The drawing under review shows one solid part. Ordinate dimensions are in mm from its lowest x, y, z. Coordinates: 2 decimals unless noted, no trailing zeros. Order: outer loops, then holes, each group sorted by start corner. A loop starts at its lowest first (then second) coordinate and runs counter-clockwise, first axis right, second up. Notation, with made-up numbers: M 47.5,-18.5 L 79.5,-18.5 A14 cw 79.5,-7.5 Z; hole C 12,44 d3. An arc over 180 degrees is marked long. Answer as a JSON object with one key per item and string values.
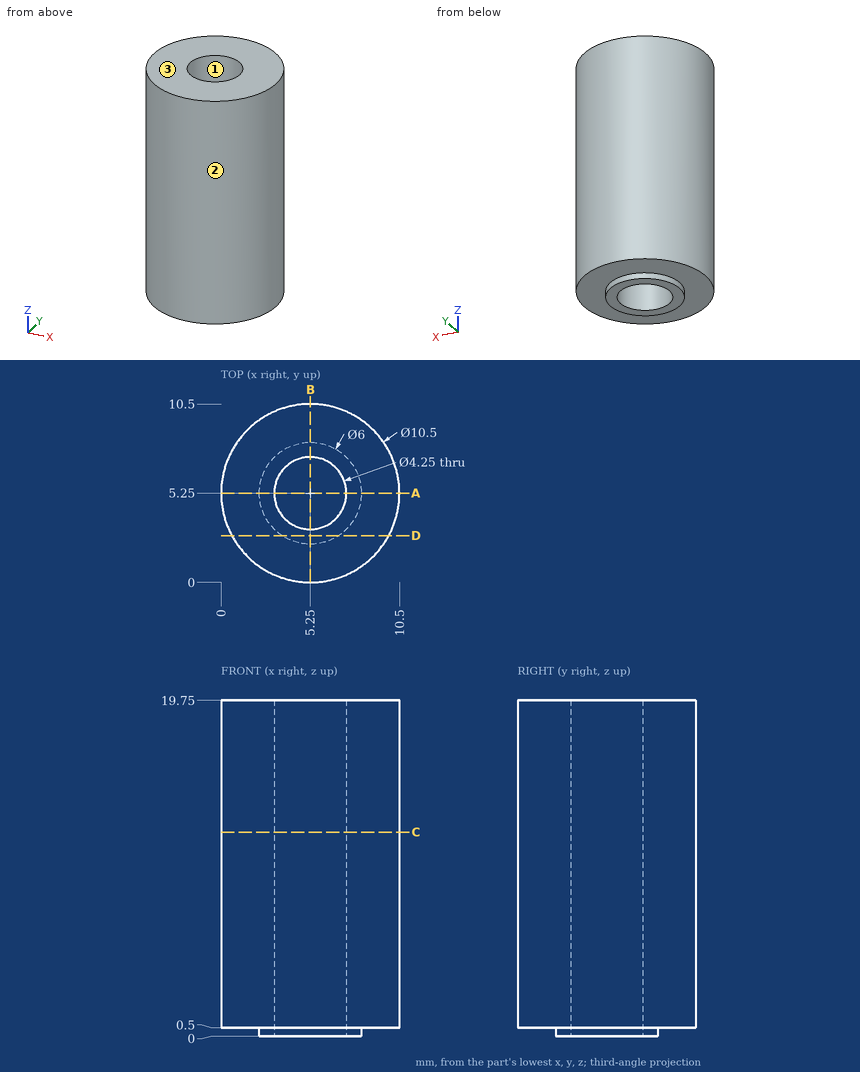
1) Add section C-C (z = 12). State the section outline as (x, y) points (3 decimals).
Taken from the geometry:
{"outline": "C 5.25,5.25 d10.5; hole C 5.25,5.25 d4.25"}
2) To check wall thickness, follow L1, parallel to Y at x = 5.25, z = 12 (3 decimals); L2, parallel to Z at x = 9.5, y = 5.5; L3, parallel to X at y = 6.25, z = 18.25 (3 decimals). State the ranges of each line that lie inside material, in increasing order.
Taken from the geometry:
{"L1": "y = 0 to 3.125, 7.375 to 10.5", "L2": "z = 0.5 to 19.75", "L3": "x = 0.096 to 3.375, 7.125 to 10.404"}
3) Insertion check: pin 1 Ø3 at (x, z) = (7, 11) entering from -Y; pin 2 Ø1.5 at (y, z) = (4, 9.5) entering from -X; pin 3 Ø1.5 at (x, z) = (3, 16) entering from +Y. Each pin has a flat end and moves straight along its axis. Give the tip position at first contact, or say it passes through.
Taken from the geometry:
{"pin 1": "stops at y = 0.01", "pin 2": "stops at x = 0.02", "pin 3": "stops at y = 10.28"}
4) Add section A-A (y = 5.25). State the section outline as (x, z) points (3 decimals), and give its area (3 significant figures).
Taken from the geometry:
{"outline": "M 0,0.5 L 2.25,0.5 L 2.25,0 L 3.125,0 L 3.125,19.75 L 0,19.75 Z; M 7.375,0 L 8.25,0 L 8.25,0.5 L 10.5,0.5 L 10.5,19.75 L 7.375,19.75 Z", "area": "121 mm2"}
5) Add section D-D (y = 2.75). State the section outline as (x, z) points.
Taken from the geometry:
{"outline": "M 0.63,0.5 L 3.59,0.5 L 3.59,0 L 6.91,0 L 6.91,0.5 L 9.87,0.5 L 9.87,19.75 L 0.63,19.75 Z"}
6) Mouldability with a two-part tool opening along Y and no side actions: class the marked faces 1, 2 and 3 as released by +Y, released by -Y, zero draft, split by the parting line, or undercut.
Taken from the geometry:
{"face 1": "undercut", "face 2": "split by the parting line", "face 3": "zero draft"}
